Here's how the part is built. I have some questions about the finished solid (model axes, mm). Face numbers are marked on the shaded views. Round coordinates to 2 decimals unless told otherwise and drop trailing zeros. Loops run counter-clockwise (first coordinate to the right, second up) from the corner with the lowest first, then second, coordinate; pieces in that order, holes last. Notation, with made-up numbers: M 42.5,-7.75 L 95.5,-7.75 A5 cw 95.5,-2.75 Z; hole C -36.5,42.25 d7. An arc over 180 degrees is marked long. One line per question, with ' | ' between items. Start each with the question number.
Autodesk Fusion 360 part; units mm, degrees
sketch "Sketch1" plane through (0, 0, 0) normal (0, 0, 1) x (1, 0, 0)
  line L0 (0, 0) -> (76.6, 0)
  line L1 (76.6, 0) -> (76.6, 156.7)
  line L2 (76.6, 156.7) -> (0, 156.7)
  line L3 (0, 156.7) -> (0, 0)
  dimension "d5" = 76.6
  dimension "d6" = 156.7
extrude "Extrude1" add sketch "Sketch1" along normal blind 2.5
sketch "Sketch2" plane through (0, 0, 2.5) normal (0, 0, 1) x (-1, 0, 0)
  line L0 (0, -156.7) -> (0, 0)
  line L1 (0, 0) -> (-76.6, 0)
  line L2 (-76.6, 0) -> (-76.6, -156.7)
  line L3 (-76.6, -156.7) -> (0, -156.7)
  line L4 (-2.5, -154.2) -> (-74.1, -154.2)
  line L5 (-74.1, -154.2) -> (-74.1, -2.5)
  line L6 (-74.1, -2.5) -> (-2.5, -2.5)
  line L7 (-2.5, -2.5) -> (-2.5, -154.2)
  dimension "d13" = 2.5
  dimension "d14" = 2.5
  dimension "d15" = 2.5
  dimension "d16" = 2.5
extrude "Extrude2" add sketch "Sketch2" along normal blind 7.25
fillet "Fillet1" radius 2 4 edges at (74.1, 154.2, 6.125) (2.5, 154.2, 6.125) (74.1, 2.5, 6.125) (2.5, 2.5, 6.125)
fillet "Fillet2" radius 2 4 edges at (0, 0, 4.875) (0, 156.7, 4.875) (76.6, 0, 4.875) (76.6, 156.7, 4.875)
sketch "Sketch3" plane through (0, 0, 2.5) normal (0, 0, 1) x (-1, 0, 0)
  arc A0 (-2.5, -4.5) -> (-4.5, -2.5) centre (-4.5, -4.5) ccw
  line L0 (-4.5, -2.5) -> (-72.1, -2.5)
  arc A1 (-72.1, -2.5) -> (-74.1, -4.5) centre (-72.1, -4.5) ccw
  line L1 (-74.1, -4.5) -> (-74.1, -152.2)
  arc A2 (-74.1, -152.2) -> (-72.1, -154.2) centre (-72.1, -152.2) ccw
  line L2 (-72.1, -154.2) -> (-4.5, -154.2)
  arc A3 (-4.5, -154.2) -> (-2.5, -152.2) centre (-4.5, -152.2) ccw
  line L3 (-2.5, -152.2) -> (-2.5, -4.5)
  line L4 (-10.5, -146.2) -> (-47.55, -146.2)
  line L5 (-47.55, -146.2) -> (-47.55, -131.2)
  line L6 (-47.55, -131.2) -> (-10.5, -131.2)
  line L7 (-10.5, -131.2) -> (-10.5, -146.2)
  dimension "d28" = 37.05
  dimension "d29" = 15
  dimension "d30" = 37.05
  dimension "d31" = 8
  dimension "d32" = 8
extrude "Extrude3" cut sketch "Sketch3" against normal blind 10 contours L4 L5 L6 L7
fillet "Fillet3" radius 2 4 edges at (10.5, 146.2, 1.25) (47.55, 146.2, 1.25) (47.55, 131.2, 1.25) (10.5, 131.2, 1.25)
sketch "Sketch4" plane through (0, 0, 0) normal (0, -1, 0) x (1, 0, 0)
  line L0 (74.6, 0) -> (74.6, 9.75)
  line L1 (74.6, 9.75) -> (2, 9.75)
  line L2 (2, 9.75) -> (2, 0)
  line L3 (2, 0) -> (74.6, 0)
  line L4 (34.88, 7.405) -> (43.22, 7.405)
  line L5 (43.22, 7.405) -> (43.22, 4.845)
  line L6 (43.22, 4.845) -> (34.88, 4.845)
  line L7 (34.88, 4.845) -> (34.88, 7.405)
  dimension "d39" = 8.34
  dimension "d40" = 2.56
  dimension "d41" = 32.88
  dimension "d42" = 2.345
extrude "Extrude4" cut sketch "Sketch4" against normal blind 7 contours L4 L5 L6 L7
fillet "Fillet4" radius 0.3 4 edges at (43.22, 1.25, 7.405) (34.88, 1.25, 7.405) (34.88, 1.25, 4.845) (43.22, 1.25, 4.845)
sketch "Sketch5" plane through (0, 0, 0) normal (0, -1, 0) x (1, 0, 0)
  line L0 (43.22, 7.105) -> (43.22, 5.145)
  arc A0 (42.92, 4.845) -> (43.22, 5.145) centre (42.92, 5.145) ccw
  line L1 (42.92, 4.845) -> (35.18, 4.845)
  arc A1 (34.88, 5.145) -> (35.18, 4.845) centre (35.18, 5.145) ccw
  line L2 (34.88, 5.145) -> (34.88, 7.105)
  arc A2 (35.18, 7.405) -> (34.88, 7.105) centre (35.18, 7.105) ccw
  line L3 (35.18, 7.405) -> (42.92, 7.405)
  arc A3 (43.22, 7.105) -> (42.92, 7.405) centre (42.92, 7.105) ccw
  line L4 (74.6, 0) -> (74.6, 9.75)
  line L5 (74.6, 9.75) -> (2, 9.75)
  line L6 (2, 9.75) -> (2, 0)
  line L7 (2, 0) -> (74.6, 0)
  circle A4 centre (64.1, 6.125) radius 2.5
  dimension "d50" = 5
  dimension "d51" = 10.5
  dimension "d52" = 3.625
extrude "Extrude5" cut sketch "Sketch5" against normal blind 6 contours A4
sketch "Sketch6" plane through (76.6, 0, 0) normal (1, 0, 0) x (0, 1, 0)
  line L0 (154.7, 0) -> (154.7, 9.75)
  line L1 (154.7, 9.75) -> (2, 9.75)
  line L2 (2, 9.75) -> (2, 0)
  line L3 (2, 0) -> (154.7, 0)
  line L4 (93.3, 7.125) -> (103.3, 7.125)
  line L5 (103.3, 7.125) -> (103.3, 5.125)
  line L6 (103.3, 5.125) -> (93.3, 5.125)
  line L7 (93.3, 5.125) -> (93.3, 7.125)
  dimension "d58" = 10
  dimension "d59" = 2
  dimension "d60" = 51.4
  dimension "d61" = 2.625
extrude "Extrude6" cut sketch "Sketch6" against normal blind 4 contours L4 L5 L6 L7
sketch "Sketch7" plane through (0, 0, 0) normal (-1, 0, 0) x (0, -1, 0)
  line L0 (-154.7, 9.75) -> (-154.7, 0)
  line L1 (-154.7, 0) -> (-2, 0)
  line L2 (-2, 0) -> (-2, 9.75)
  line L3 (-2, 9.75) -> (-154.7, 9.75)
  line L4 (-137.7, 7.125) -> (-122.7, 7.125)
  line L5 (-122.7, 7.125) -> (-122.7, 5.125)
  line L6 (-122.7, 5.125) -> (-137.7, 5.125)
  line L7 (-137.7, 5.125) -> (-137.7, 7.125)
  dimension "d70" = 15
  dimension "d71" = 2
  dimension "d72" = 17
  dimension "d73" = 2.625
extrude "Extrude7" cut sketch "Sketch7" against normal blind 7 contours L4 L5 L6 L7
sketch "Sketch8" plane through (0, 0, 0) normal (-1, 0, 0) x (0, -1, 0)
  line L0 (-122.7, 7.125) -> (-122.7, 5.125)
  line L1 (-122.7, 5.125) -> (-137.7, 5.125)
  line L2 (-137.7, 5.125) -> (-137.7, 7.125)
  line L3 (-137.7, 7.125) -> (-122.7, 7.125)
  line L4 (-154.7, 9.75) -> (-154.7, 0)
  line L5 (-154.7, 0) -> (-2, 0)
  line L6 (-2, 0) -> (-2, 9.75)
  line L7 (-2, 9.75) -> (-154.7, 9.75)
  line L8 (-104.7, 7.125) -> (-79.7, 7.125)
  line L9 (-79.7, 7.125) -> (-79.7, 5.125)
  line L10 (-79.7, 5.125) -> (-104.7, 5.125)
  line L11 (-104.7, 5.125) -> (-104.7, 7.125)
  dimension "d76" = 25
  dimension "d77" = 2
  dimension "d78" = 18
  dimension "d79" = 2.625
extrude "Extrude8" cut sketch "Sketch8" against normal blind 5 contours L8 L9 L10 L11
fillet "Fillet5" radius 0.4 4 edges at (1.25, 122.7, 7.125) (1.25, 122.7, 5.125) (1.25, 137.7, 5.125) (1.25, 137.7, 7.125)
fillet "Fillet6" radius 0.4 4 edges at (1.25, 104.7, 7.125) (1.25, 104.7, 5.125) (1.25, 79.7, 7.125) (1.25, 79.7, 5.125)
fillet "Fillet7" radius 0.4 4 edges at (75.35, 93.3, 5.125) (75.35, 103.3, 7.125) (75.35, 103.3, 5.125) (75.35, 93.3, 7.125)
equation "phone_height = 154.2 mm"
equation "phone_width = 74.1 mm"
equation "phone_depth = 7.25 mm"
equation "case_depth = 2.5 mm"
equation "d5 = phone_width + case_depth"
equation "d6 = phone_height + case_depth"
equation "d11 = case_depth"
equation "d13 = case_depth"
equation "d14 = case_depth"
equation "d15 = case_depth"
equation "d16 = case_depth"
equation "d17 = phone_depth"
equation "fillet_amount = 2 mm"
equation "d21 = fillet_amount"
equation "d23 = fillet_amount"
equation "camera_margin_top = 8 mm"
equation "camera_margin_left = 8 mm"
equation "camera_height = 15 mm"
equation "camera_width = phone_width * 0.5"
equation "d28 = camera_width"
equation "d29 = camera_height"
equation "d31 = camera_margin_left"
equation "d32 = camera_margin_top"
equation "d36 = fillet_amount"
equation "usbc_width = 8.34 mm"
equation "usbc_height = 2.56 mm"
equation "d39 = usbc_width"
equation "d40 = usbc_height"
equation "d41 = ( phone_width / 2 ) - ( usbc_width / 2 )"
equation "d42 = ( phone_depth / 2 ) - ( usbc_height / 2 )"
equation "d46 = usb_c_fillet"
equation "usb_c_fillet = 0.3 mm"
equation "aux_diameter = 5 mm"
equation "aux_margin_right = 8 mm"
equation "d50 = aux_diameter"
equation "d51 = aux_margin_right + ( aux_diameter / 2 )"
equation "d52 = phone_depth / 2"
equation "sidebutton_width = 10 mm"
equation "sidebutton_height = 2 mm"
equation "sidebutton_margin_right = phone_height / 3"
equation "d58 = sidebutton_width"
equation "d59 = sidebutton_height"
equation "d60 = sidebutton_margin_right"
equation "d61 = ( phone_depth / 2 ) - ( sidebutton_height / 2 )"
equation "volume_width = 25 mm"
equation "volume_height = 2 mm"
equation "sliderbutton_width = 15 mm"
equation "sliderbutton_height = 2 mm"
equation "sliderbutton_margin_left = 17 mm"
equation "volumebutton_distance_to_sliderbutton = 18 mm"
equation "d70 = sliderbutton_width"
equation "d71 = sliderbutton_height"
equation "d72 = sliderbutton_margin_left"
equation "d73 = ( phone_depth / 2 ) - ( sliderbutton_height / 2 )"
equation "d76 = volume_width"
equation "d77 = volume_height"
equation "d78 = volumebutton_distance_to_sliderbutton"
equation "d79 = ( phone_depth / 2 ) - ( volume_height / 2 )"
equation "button_fillet = 0.4 mm"
equation "d84 = button_fillet"
equation "d86 = button_fillet"
equation "d88 = button_fillet"
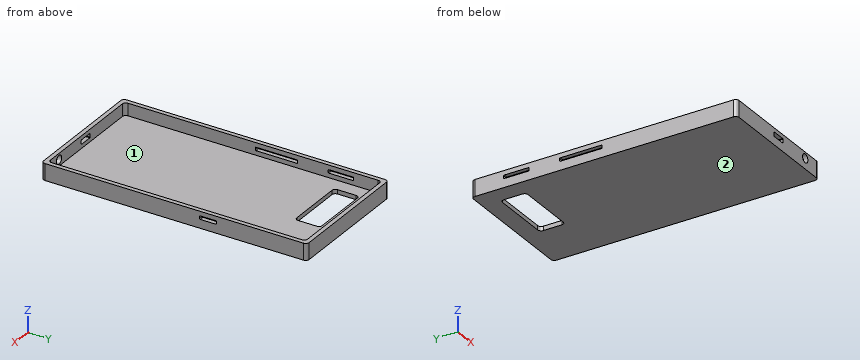
1) Imagine slicing it at C-C (x = 70.5). Write out the boundary of the cut face in (y, z), then the cut area to 3 significant figures.
2) I'm going to push flat-ended pins straight in: pin 1 Ø2 at (x, y) = (8, 101) entering from -Z; pin 2 Ø1 at (x, y) = (64, 44) entering from +Z; pin 3 Ø0.6 at (x, z) = (75, 6) entering from -Y; pin 4 Ø1.6 at (y, z) = (1, 6.5) entering from +X. Where does each tip first touch, or does it pass through?
3) Imagine slicing it at A-A (x = 26). Write out the boundary of the cut face in (y, z).
4) We'd pull the mould along Y, two halves only. Please class the marked faces 1 and 2: pulls with the +Y half, pulls with the -Y half, needs draft (parallel to the pull), parting line crosses it, or undercut.
5) Please list where these lines run through material, in increasing order: L1, parallel to Z at x = 64.1, y = 1.45 (3 decimals); L2, parallel to X at y = 25, z = 3.75; L3, parallel to Y at x = 36, z = 1. Write a range as from..to.
6) Imagine slicing it at B-B (y = 66). Write out the boundary of the cut face in (x, z).
Results are:
1) outline: M 0,0 L 156.7,0 L 156.7,9.75 L 154.2,9.75 L 154.2,2.5 L 2.5,2.5 L 2.5,9.75 L 0,9.75 Z | area: 428 mm²
2) pin 1: z = 0 | pin 2: z = 2.5 | pin 3: y = 0 | pin 4: x = 76.59
3) outline: M 0,0 L 131.2,0 L 131.2,2.5 L 2.5,2.5 L 2.5,9.75 L 0,9.75 Z; M 146.2,0 L 156.7,0 L 156.7,9.75 L 154.2,9.75 L 154.2,2.5 L 146.2,2.5 Z
4) face 1: undercut | face 2: needs draft
5) L1: 0..3.625, 8.625..9.75 | L2: 0..2.5, 74.1..76.6 | L3: 0..131.2, 146.2..156.7
6) outline: M 0,0 L 76.6,0 L 76.6,9.75 L 74.1,9.75 L 74.1,2.5 L 2.5,2.5 L 2.5,9.75 L 0,9.75 Z
